Check sheet for the drawn part. Datum: minimum x, y, z corner. Units: mm. A direction names the side the tool comes from. Coordinates: 2 decimals unless noted, no trailing zeros. Order: outer loops, then holes, each group sorted by start corner. A loop starts at its lowest first (then second) coordinate and runs counter-clockwise, first axis right, second up. Notation, with made-up numbers: (-34.5, -3.75) - (16.5, -3.75) arc R18 cw to (16.5, 23.25) - close; hole circle Ø7 at (71, 20). An arc over 180 degrees is marked (long way). Answer as CSV lines item,"result". Start each with the question number.
1. Section check C-C (x = 0.5). Record the cut outline in (y, z).
2. Section check B-B (y = 1). Record the cut outline in (x, z), and give its area (3 significant figures).
3. Section check A-A (z = 9.25). Record the cut outline in (x, y), and give its area (3 significant figures).
4. Section check D-D (y = 1.6). Record the cut outline in (x, z).
5. Go/stop test with flat-tipped pins: pin 1 (1.1 mm diameter, centred on x = 2.5, z = 8.5, fed in from -Y); pin 2 (0.8 mm diameter, centred on y = 1, z = 8, fed in from +X); pin 3 (0.8 mm diameter, centred on x = 1, z = 7.5, fed in from +Y). Record where each tip stops, or that it passes through.
6. Material ranges on L1, parallel to X at y = 1.15, z = 10.25; L2, parallel to Y at x = 0.6, z = 5; L3, parallel to Z at x = 2.3, y = 1.65, recorded low to high. Write a range as [from, to].
7. Set-up check for the marked faces 1, 2 and 3: record each of +Z, -Z, +X, -X, +Y, -Y from which the full face is reachable in a straight line by a thin tool's end or side.
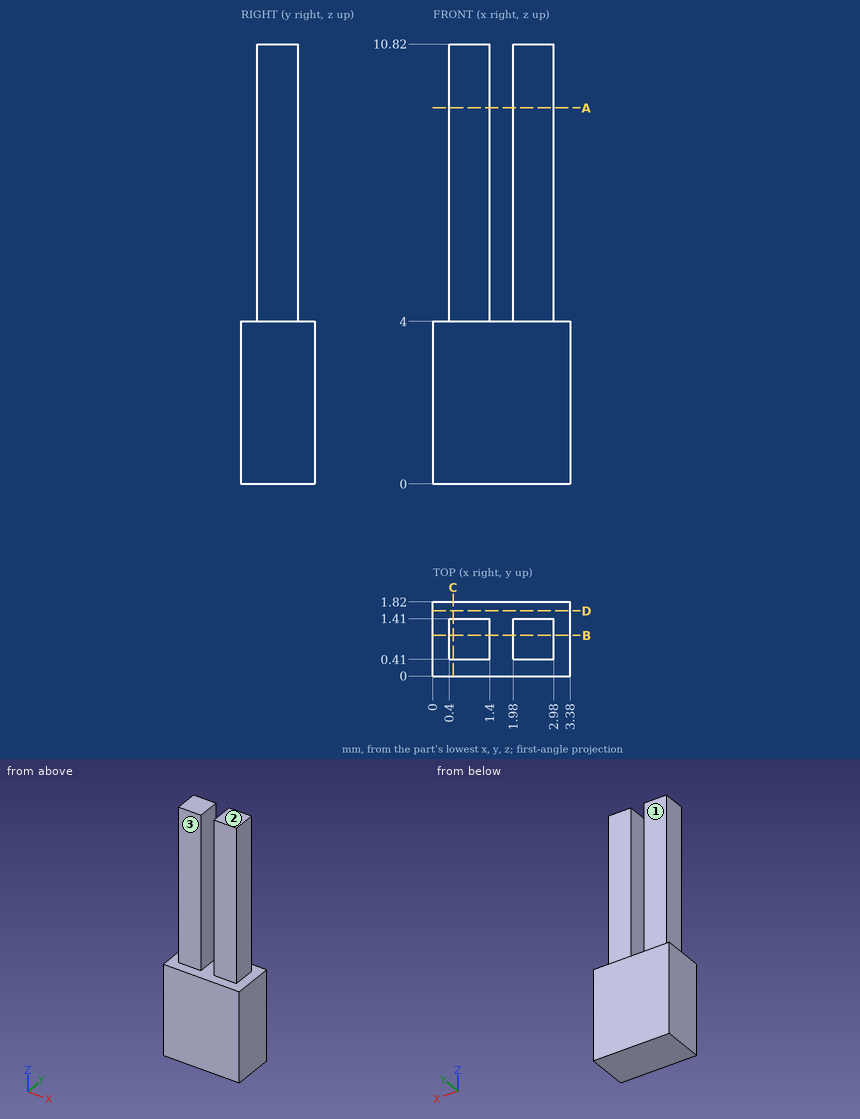
Evaluation:
1,outline,"(0, 0) - (1.82, 0) - (1.82, 4) - (1.41, 4) - (1.41, 10.82) - (0.41, 10.82) - (0.41, 4) - (0, 4) - close"
2,outline,"(0, 0) - (3.38, 0) - (3.38, 4) - (2.98, 4) - (2.98, 10.82) - (1.98, 10.82) - (1.98, 4) - (1.4, 4) - (1.4, 10.82) - (0.4, 10.82) - (0.4, 4) - (0, 4) - close"
2,area,"27.2 mm²"
3,outline,"(0.4, 0.41) - (1.4, 0.41) - (1.4, 1.41) - (0.4, 1.41) - close; (1.98, 0.41) - (2.98, 0.41) - (2.98, 1.41) - (1.98, 1.41) - close"
3,area,"2.00 mm²"
4,outline,"(0, 0) - (3.38, 0) - (3.38, 4) - (0, 4) - close"
5,pin 1,"stops at y = 0.41"
5,pin 2,"stops at x = 2.98"
5,pin 3,"stops at y = 1.41"
6,L1,"x = [0.4, 1.4], [1.98, 2.98]"
6,L2,"y = [0.41, 1.41]"
6,L3,"z = [0, 4]"
7,face 1,"+Z, +X, -X, +Y"
7,face 2,"+Z, +X, -X, +Y, -Y"
7,face 3,"+Z, +X, -X, -Y"
